The listing builds one solid part. Answer for the finished solid, in the listing's coordinates (mm). Give positions to 0.01 mm unless a question says otherwise; leave off trailing zeros. Loops run counter-clockwise (first coordinate to the right, second up) from the corner with the lowest first, then second, coordinate; pieces in that order, holes last. Notation, with made-up numbers: M 40,4.5 L 69,4.5 A12 cw 69,19.5 Z; hole C 6.5,-22 d8. An arc over 180 degrees is marked long. Use one line per item in the form item = value. Start each with the question number.
1. The part is cut by section A-A (x = -27.4). Write down the section's boundary in (y, z), and give its area (3 significant figures).
2. The part is cut by section C-C (z = 1.25). Give the number of separate pieces and of enclosed holes in the cut face, and give its area (3 significant figures).
3. The part is cut by section B-B (y = 28.28). Write down the section's boundary in (x, z).
4. Straight lines are drawn through the part: line 1 (Y direction, x = -27.4, z = 0.6); line 2 (Y direction, x = -39.88, z = 0.9); line 3 (X direction, y = -12, z = 0.75). For each, find the intervals that lie inside material, in ascending order. Write a range as from..to.
5. The part is cut by section D-D (x = -39.88). Write down the section's boundary in (y, z), and give its area (3 significant figures).
6. Each of these flat-tipped pins is pushed along its axis until it touches: pin 1 Ø4.5 at (x, y) = (-27.4, 14.89) entering from -Z; pin 2 Ø1 at (x, z) = (33.5, 1) entering from +Y. Where does it stop, or does it pass through?
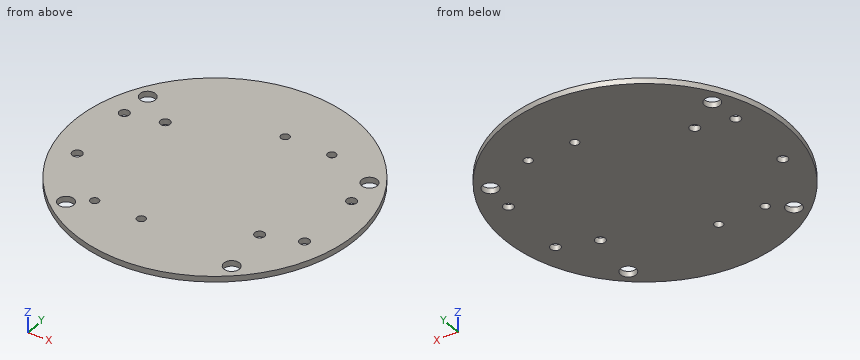
from build123d import *

# Parameters (mm, degrees)
ESBO_O1_R                = 50
RESSALTO_EXTRUS_O1_DEPTH = 2
ESBO_O2_R                = 2.75
CORTE_EXTRUS_O1_DEPTH    = 2
ESBO_O3_R                = 1.75
ESBO_O3_R_2              = 1.5
CORTE_EXTRUS_O2_DEPTH    = 10


with BuildPart() as part:
    # Esboço1 → Ressalto-extrusão1 (new body)
    with BuildSketch(Plane.XY):
        Circle(ESBO_O1_R)
    extrude(amount=RESSALTO_EXTRUS_O1_DEPTH)

    # Esboço2 → Corte-extrusão1 (cut)
    with BuildSketch(Plane.XY.offset(2)):
        with Locations((-29, -34.409301068)):
            Circle(ESBO_O2_R)
        with Locations((29, -34.409301068)):
            Circle(ESBO_O2_R)
        with Locations((-38.824197531, 22.752619324)):
            Circle(ESBO_O2_R)
        with Locations((38.824197531, 22.752619324)):
            Circle(ESBO_O2_R)
    extrude(amount=-CORTE_EXTRUS_O1_DEPTH, mode=Mode.SUBTRACT)

    # Esboço3 → Corte-extrusão2 (cut)
    with BuildSketch(Plane.XY.offset(2)):
        with Locations((-27.4, 14.89)):
            Circle(ESBO_O3_R)
        with Locations((26.91, -16.73)):
            Circle(ESBO_O3_R)
        with Locations((-39.88, -12.4)):
            Circle(ESBO_O3_R)
        with Locations((-39.88, 12.11)):
            Circle(ESBO_O3_R)
        with Locations((39.68, 12.16)):
            Circle(ESBO_O3_R)
        with Locations((39.68, -12.34)):
            Circle(ESBO_O3_R)
        with Locations((5.59, 28.28)):
            Circle(ESBO_O3_R_2)
        with Locations((21.91, 28.28)):
            Circle(ESBO_O3_R_2)
        with Locations((-6.08, -29.3)):
            Circle(ESBO_O3_R_2)
        with Locations((-22.4, -29.3)):
            Circle(ESBO_O3_R_2)
    extrude(amount=-CORTE_EXTRUS_O2_DEPTH, mode=Mode.SUBTRACT)


solid = part.part
Derived:
q1.outline = M -41.82,0 L -36.65,0 L -36.65,2 L -41.82,2 Z; M -32.17,0 L 13.14,0 L 13.14,2 L -32.17,2 Z; M 16.64,0 L 41.82,0 L 41.82,2 L 16.64,2 Z
q1.area = 151 mm2
q2.separate_pieces = 1
q2.enclosed_holes = 14
q2.area = 7,670 mm2
q3.outline = M -41.23,0 L 4.09,0 L 4.09,2 L -41.23,2 Z; M 7.09,0 L 20.41,0 L 20.41,2 L 7.09,2 Z; M 23.41,0 L 41.23,0 L 41.23,2 L 23.41,2 Z
q4.line_1 = -41.82..-36.65, -32.17..13.14, 16.64..41.82
q4.line_2 = -30.16..-14.15, -10.65..10.36, 13.86..20.21, 25.29..30.16
q4.line_3 = -48.54..-41.58, -38.18..37.96, 41.4..48.54
q5.outline = M -30.16,0 L -14.15,0 L -14.15,2 L -30.16,2 Z; M -10.65,0 L 10.36,0 L 10.36,2 L -10.65,2 Z; M 13.86,0 L 20.21,0 L 20.21,2 L 13.86,2 Z; M 25.29,0 L 30.16,0 L 30.16,2 L 25.29,2 Z
q5.area = 96.5 mm2
q6.pin_1 = 0
q6.pin_2 = 37.56
